Input: part model. Units: mm. Frame: model coordinates. Coordinates: 2 decimals unless noted, no trailing zeros. Order: outer loops, then holes, each group sorted by start corner. A loop starts at its lowest first (then second) coordinate and runs counter-clockwise, first axis right, second up.
from build123d import *

# Parameters (mm, degrees)
ESQUISSE1_W             = 32
ESQUISSE1_H             = 6
BOSS_EXTRU_1_DEPTH      = 6
ESQUISSE2_R             = 0.625
ENL_V_MAT_EXTRU_1_DEPTH = 34.105890714
ESQUISSE3_R             = 0.625
ENL_V_MAT_EXTRU_2_DEPTH = 34.105890714


with BuildPart() as part:
    # Esquisse1 → Boss.-Extru.1 (new body)
    with BuildSketch(Plane.XY):
        with Locations((16, 3)):
            Rectangle(ESQUISSE1_W, ESQUISSE1_H)
    extrude(amount=BOSS_EXTRU_1_DEPTH)

    # Esquisse2 → Enlèv. mat.-Extru.1 (cut, through all)
    with BuildSketch(Plane(origin=(32, 0, 0), x_dir=(0, 0, -1), z_dir=(1, 0, 0))):
        with Locations((-2, 3)):
            Circle(ESQUISSE2_R)
    extrude(amount=-ENL_V_MAT_EXTRU_1_DEPTH, mode=Mode.SUBTRACT)

    # Esquisse3 → Enlèv. mat.-Extru.2 (cut, through all)
    with BuildSketch(Plane(origin=(0, 6, 0), x_dir=(1, 0, 0), z_dir=(0, 1, 0))):
        with Locations(Location((29.5, -4, 0), (0, 0, 180))):
            Circle(ESQUISSE3_R)
        with Locations(Location((2.5, -4, 0), (0, 0, 180))):
            Circle(ESQUISSE3_R)
    extrude(amount=-ENL_V_MAT_EXTRU_2_DEPTH, mode=Mode.SUBTRACT)


solid = part.part
Item 1: Draft query along Y for faces 1 (the face through (16, 6, 3)), 2 (the face through (16, 0, 3)), 3 (the face through (16.22, 2.39, 2.14)), 4 (the face through (28.904, 3.042, 4.188)). Return one class per face: pulls with the +Y half, pulls with the -Y half, needs draft (parallel to the pull), parting line crosses it, or undercut.
Response values:
face 1: pulls with the +Y half
face 2: pulls with the -Y half
face 3: undercut
face 4: needs draft
Item 2: Ray query, probe 1 along Y at (x, z) = (9.5, 2) (3 decimals); probe 2 along X at (y, z) = (3.25, 3.6); probe 3 along Y at (x, z) = (19, 2.5) (3 decimals). Return the intervals inside material, ascending.
Response values:
probe 1: y = 0 to 2.375, 3.625 to 6
probe 2: x = 0 to 2.02, 2.98 to 29.02, 29.98 to 32
probe 3: y = 0 to 2.625, 3.375 to 6
Item 3: Cut plane A-A on x = 2.5. Return loops of the section in (y, z) (3 decimals).
Response values:
outline: (0, 0) - (6, 0) - (6, 3.375) - (0, 3.375) - close; (0, 4.625) - (6, 4.625) - (6, 6) - (0, 6) - close; hole circle Ø1.25 at (3, 2)
Item 4: Cut plane B-B on z = 4. Return loops of the section in (x, y) (3 decimals), then the cut area to 3 significant figures.
Response values:
outline: (0, 0) - (1.875, 0) - (1.875, 6) - (0, 6) - close; (3.125, 0) - (28.875, 0) - (28.875, 6) - (3.125, 6) - close; (30.125, 0) - (32, 0) - (32, 6) - (30.125, 6) - close
area: 177 mm2
Item 5: Cut plane C-C on z = 2. Return loops of the section in (x, y) (3 decimals).
Response values:
outline: (0, 0) - (32, 0) - (32, 2.375) - (0, 2.375) - close; (0, 3.625) - (32, 3.625) - (32, 6) - (0, 6) - close
Item 6: Pin query (flat end, axial travel): pin 1 Ø1 at (y, z) = (3, 2) entering from +X. Return the tip coordinate at first contact, or that it passes through.
Response values:
pin 1: passes through
